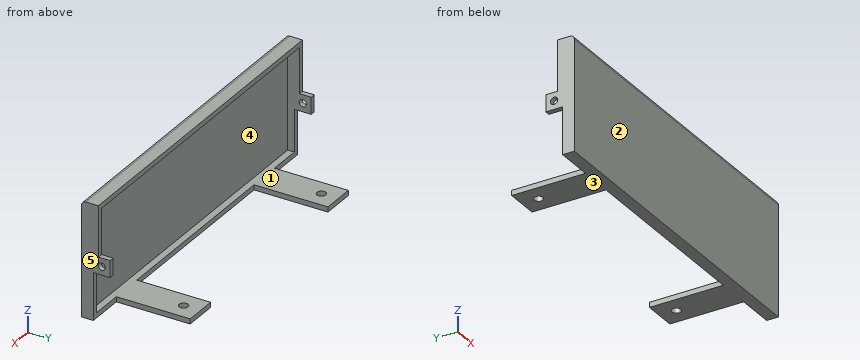
Autodesk Fusion 360 part; units mm, degrees
sketch "스케치1" plane through (0, 0, 0) normal (1, 0, 0) x (0, 1, 0)
  line L0 (0, 0) -> (-7, 0)
  line L1 (-7, 0) -> (-7, 68)
  line L2 (-7, 68) -> (0, 68)
  line L3 (0, 68) -> (0, 0)
  line L4 (0, 0) -> (-4, 0)
  line L5 (-4, 0) -> (-4, 68)
  line L6 (-4, 68) -> (0, 68)
  line L7 (0, 68) -> (0, 0)
  dimension "d1" = 7
  dimension "d2" = 68
  dimension "d3" = 4
extrude "돌출1" add sketch "스케치1" along normal blind 200
sketch "스케치2" plane through (0, 0, 0) normal (0, 1, 0) x (-1, 0, 0)
  line L0 (0, 0) -> (0, 68)
  line L1 (0, 68) -> (-200, 68)
  line L2 (-200, 68) -> (-200, 0)
  line L3 (-200, 0) -> (0, 0)
  line L4 (-200, 68) -> (-197, 68)
  line L5 (-197, 68) -> (-197, 65)
  line L6 (-197, 65) -> (-200, 65)
  line L7 (-200, 65) -> (-200, 68)
  line L8 (0, 0) -> (-3, 0)
  line L9 (-3, 0) -> (-3, 3)
  line L10 (-3, 3) -> (0, 3)
  line L11 (0, 3) -> (0, 0)
  line L12 (-3, 3) -> (-197, 3)
  line L13 (-197, 3) -> (-197, 65)
  line L14 (-197, 65) -> (-3, 65)
  line L15 (-3, 65) -> (-3, 3)
  dimension "d6" = 3
  dimension "d7" = 3
  dimension "d8" = 3
extrude "돌출2" cut sketch "스케치2" against normal blind 4 contours L12 L13 L14 L15
sketch "스케치3" plane through (0, 0, 0) normal (0, 1, 0) x (-1, 0, 0)
  line L0 (-197, 3) -> (-197, 65)
  line L1 (-197, 65) -> (-3, 65)
  line L2 (-3, 65) -> (-3, 3)
  line L3 (-3, 3) -> (-197, 3)
  line L4 (0, 0) -> (0, 68)
  line L5 (0, 68) -> (-200, 68)
  line L6 (-200, 68) -> (-200, 0)
  line L7 (-200, 0) -> (0, 0)
  line L8 (-197, 3) -> (-177.5, 3)
  line L9 (-177.5, 3) -> (-157.5, 3)
  line L10 (-157.5, 3) -> (-157.5, 0)
  line L11 (-157.5, 0) -> (-177.5, 0)
  line L12 (-177.5, 0) -> (-177.5, 3)
  line L13 (-3, 3) -> (-22.5, 3)
  line L14 (-22.5, 3) -> (-42.5, 3)
  line L15 (-42.5, 3) -> (-42.5, 0)
  line L16 (-42.5, 0) -> (-22.5, 0)
  line L17 (-22.5, 0) -> (-22.5, 3)
  dimension "d11" = 19.5
  dimension "d12" = 20
  dimension "d13" = 19.5
  dimension "d14" = 20
  dimension "d15" = 3
extrude "돌출3" add sketch "스케치3" along normal blind 44 contours L3 L7 L9 L10 L11 L12 | L3 L7 L14 L15 L16 L17
sketch "스케치4" plane through (0, 0, 3) normal (0, 0, 1) x (-1, 0, 0)
  line L0 (-22.5, 0) -> (-3, 0)
  line L1 (-3, 0) -> (-3, 4)
  line L2 (-3, 4) -> (-197, 4)
  line L3 (-197, 4) -> (-197, 0)
  line L4 (-197, 0) -> (-177.5, 0)
  line L5 (-177.5, 0) -> (-177.5, -44)
  line L6 (-177.5, -44) -> (-157.5, -44)
  line L7 (-157.5, -44) -> (-157.5, 0)
  line L8 (-157.5, 0) -> (-42.5, 0)
  line L9 (-42.5, 0) -> (-42.5, -44)
  line L10 (-42.5, -44) -> (-22.5, -44)
  line L11 (-22.5, -44) -> (-22.5, 0)
  line L12 (-177.5, -44) -> (-167.5, -44)
  line L13 (-167.5, -44) -> (-167.5, -34)
  line L14 (-167.5, -34) -> (-177.5, -34)
  line L15 (-177.5, -34) -> (-177.5, -44)
  line L16 (-42.5, -44) -> (-32.5, -44)
  line L17 (-32.5, -44) -> (-32.5, -34)
  line L18 (-32.5, -34) -> (-42.5, -34)
  line L19 (-42.5, -34) -> (-42.5, -44)
  circle A0 centre (-167.5, -34) radius 2.65
  circle A1 centre (-32.5, -34) radius 2.65
  dimension "d18" = 10
  dimension "d19" = 10
  dimension "d20" = 10
  dimension "d21" = 10
  dimension "d22" = 5.3
  dimension "d23" = 5.3
extrude "돌출4" cut sketch "스케치4" against normal blind 3 contours L17 L18 A1 | L17 L18 A1 | L13 L14 A0 | L13 L14 A0
fillet "필렛1" radius 2.5 1 edges at (100, -7, 68)
sketch "스케치5" plane through (0, 0, 0) normal (0, 1, 0) x (-1, 0, 0)
  line L0 (-177.5, 0) -> (-177.5, 3)
  line L1 (-177.5, 3) -> (-197, 3)
  line L2 (-197, 3) -> (-197, 65)
  line L3 (-197, 65) -> (-3, 65)
  line L4 (-3, 65) -> (-3, 3)
  line L5 (-3, 3) -> (-22.5, 3)
  line L6 (-22.5, 3) -> (-22.5, 0)
  line L7 (-22.5, 0) -> (0, 0)
  line L8 (0, 0) -> (0, 68)
  line L9 (0, 68) -> (-200, 68)
  line L10 (-200, 68) -> (-200, 0)
  line L11 (-200, 0) -> (-177.5, 0)
  line L12 (-197, 3) -> (-200, 3)
  line L13 (-200, 3) -> (-200, 38)
  line L14 (-200, 38) -> (-197, 38)
  line L15 (-197, 38) -> (-197, 3)
  line L16 (-200, 38) -> (-197, 38)
  line L17 (-197, 38) -> (-197, 28)
  line L18 (-197, 28) -> (-200, 28)
  line L19 (-200, 28) -> (-200, 38)
  line L20 (-3, 3) -> (0, 3)
  line L21 (0, 3) -> (0, 38)
  line L22 (0, 38) -> (-3, 38)
  line L23 (-3, 38) -> (-3, 3)
  line L24 (0, 38) -> (-3, 38)
  line L25 (-3, 38) -> (-3, 28)
  line L26 (-3, 28) -> (0, 28)
  line L27 (0, 28) -> (0, 38)
  dimension "d28" = 3
  dimension "d29" = 35
  dimension "d30" = 10
  dimension "d31" = 35
  dimension "d32" = 10
extrude "돌출5" add sketch "스케치5" along normal blind 10 contours L2 L10 L13 L14 L15 L16 L17 L18 L19 | L4 L8 L21 L22 L23 L24 L25 L26 L27
sketch "스케치6" plane through (200, 0, 0) normal (1, 0, 0) x (0, 1, 0)
  arc A0 (-4.5, 68) -> (-7, 65.5) centre (-4.5, 65.5) ccw
  line L0 (-7, 65.5) -> (-7, 0)
  line L1 (-7, 0) -> (0, 0)
  line L2 (0, 0) -> (0, 28)
  line L3 (0, 28) -> (10, 28)
  line L4 (10, 28) -> (10, 38)
  line L5 (10, 38) -> (0, 38)
  line L6 (0, 38) -> (0, 68)
  line L7 (0, 68) -> (-4.5, 68)
  line L8 (10, 38) -> (5, 38)
  line L9 (5, 38) -> (5, 33)
  line L10 (5, 33) -> (10, 33)
  line L11 (10, 33) -> (10, 38)
  circle A1 centre (5, 33) radius 2.15
  dimension "d35" = 5
  dimension "d36" = 5
  dimension "d37" = 4.3
extrude "돌출6" cut sketch "스케치6" against normal blind 260 contours L9 L10 A1 | L9 L10 A1
extrude "돌출7" add 1 faces at (67.6667, 0, 67) along direction (0, 1, 0) blind 3
Can you work these out from the model? Positions are in its coordinate system, mm. Face numbers are marked on the shaded views. A direction names the side the tool comes from. Round coordinates to 2 decimals unless told otherwise and drop trailing zeros. Order: outer loops, then holes, each group sorted by start corner. A loop starts at its lowest first (then second) coordinate and runs counter-clockwise, first axis right, second up. Notation, with made-up numbers: M 73.25,13.5 L 109.25,13.5 A19 ccw 109.25,33.5 Z; hole C 33,-21 d3. An arc over 180 degrees is marked long. Use a Markdown table: item, result.
1) If we mould it in two halves opening along Z, with no side actions, what happens to the marked faces 3, 4 and 5? For each: +Z half, -Z half, draft (parallel to the pull), parting line (faces both ways), or undercut.
Geometry says:
| item | result |
|---|---|
| face 3 | -Z half |
| face 4 | undercut |
| face 5 | draft |
2) Imagine slicing it at C-C (x = 53). List the corners of the cut face in (y, z) for me, then the cut area to 3 significant figures.
Geometry says:
| item | result |
|---|---|
| outline | M -7,0 L 0,0 L 0,3 L -4,3 L -4,65 L 3,65 L 3,68 L -4.5,68 A2.5 ccw -7,65.5 Z |
| area | 236 mm² |
3) On a 3-axis mill with a long thin cutter (end or side, diameter ignored), from which of +Z, -Z, +X, -X, +Y, -Y can I reach the whole of each face in a straight line? I mean the marked faces 1 and 2. Say none if no direction works.
Geometry says:
| item | result |
|---|---|
| face 1 | +Y |
| face 2 | +Z, -Z, +X, -X, -Y |
4) Imagine slicing it at D-D (z = 41). List the corners of the cut face in (x, y) for me, then the cut area to 3 significant figures.
Geometry says:
| item | result |
|---|---|
| outline | M 0,-7 L 200,-7 L 200,3 L 197,3 L 197,-4 L 3,-4 L 3,3 L 0,3 Z |
| area | 642 mm² |
5) Imagine slicing it at B-B (z = 33). List the corners of the cut face in (x, y) for me, then the cut area to 3 significant figures.
Geometry says:
| item | result |
|---|---|
| outline | M 0,-7 L 200,-7 L 200,2.85 L 197,2.85 L 197,-4 L 3,-4 L 3,2.85 L 0,2.85 Z; M 0,7.15 L 3,7.15 L 3,10 L 0,10 Z; M 197,7.15 L 200,7.15 L 200,10 L 197,10 Z |
| area | 658 mm² |
6) If I drill on line 1 along X through (y, z) = (34, 1.65); line 2 along Z through (x, y) = (1.1, 5); line 3 along Y through (x, z) = (32.5, 2.05), over which ranges is the centre line in solid material (lowest first)?
Geometry says:
| item | result |
|---|---|
| line 1 | x = 22.5 to 29.85, 35.15 to 42.5, 157.5 to 164.85, 170.15 to 177.5 |
| line 2 | z = 28 to 30.85, 35.15 to 38 |
| line 3 | y = -7 to 31.35, 36.65 to 44 |
7) Imagine slicing it at A-A (y = 12). List the corners of the cut face in (x, z) for me.
Geometry says:
| item | result |
|---|---|
| outline | M 22.5,0 L 42.5,0 L 42.5,3 L 22.5,3 Z; M 157.5,0 L 177.5,0 L 177.5,3 L 157.5,3 Z |
8) I'm going to push flat-ended pins straight in: P1, Ø2.5, axis at y = 21.5, z = 1, coming from the -X side; P2, Ø7, axis at x = 184.5, z = 16, coming from the +Y side; P3, Ø11, axis at y = 0.5, z = 24, coming from the -X side; P4, Ø0.9, axis at x = 198.5, z = 35, coming from the +Y side. Where does each tip first touch, or does it pass through?
Geometry says:
| item | result |
|---|---|
| P1 | stops at x = 22.5 |
| P2 | stops at y = -4 |
| P3 | stops at x = 0 |
| P4 | stops at y = 10 |
